The listing builds one solid part. Answer for the finished solid, in the listing's coordinates (mm). Face numbers are marked on the shaded views. A direction names the side the tool comes from. Coordinates: 2 decimals unless noted, no trailing zeros. Return JSON: item names as keys, results as strings. Group by question number.
1. Each of these flat-tipped pins is pushed along its axis until it touches: P1, Ø3, axis at x = -27.5, y = -23, coming from the +Z side; P2, Ø3, axis at x = -21, z = 20.5, coming from the +Y side; P3, Ø12, axis at x = 2.5, y = -15, coming from the -Z side; P4, Ø3, axis at x = 52, z = 13.5, coming from the +Y side. Where does it stop, or does it pass through?
2. The mould has two halves that part along X. Classify the marked faces 5, 6 and 7: pulls with the +X half, pulls with the -X half, needs draft (parallel to the pull), parting line crosses it, or undercut.
3. Which of the six approach directions +Z, -Z, +X, -X, +Y, -Y give full straight-line access (tool end or side, diameter ignored) to the marked faces 1, 2, 3 and 4?
4. Find the intervals of material crossed by line 1 along X through (y, z) = (-25, 13.25); line 2 along Y through (x, z) = (0, 20.65); line 3 along Z through (x, y) = (28, -15.75), in increasing order.
5. Section B-B (z = 21) is taken. State how many separate pieces and enclosed holes the cut face has, and give its area (3 significant figures).
```python
from build123d import *
from OCP.BRepFilletAPI import BRepFilletAPI_MakeChamfer

# Parameters (mm, degrees)
SKETCH1_R           = 2.675
SKETCH1_R_2         = 6.5
BOSS_EXTRUDE1_DEPTH = 26
CUT_EXTRUDE2_START  = 6
SKETCH1_4_R         = 11.05
SKETCH1_4_R_2       = 6.5
CUT_EXTRUDE2_DEPTH  = 8
SKETCH5_R           = 11.05
CUT_EXTRUDE6_DEPTH  = 6
CUT_EXTRUDE6_DRAFT  = 5
SKETCH4_R           = 5.25
CUT_EXTRUDE5_DEPTH  = 6.5
CUT_EXTRUDE10_START = -7
SKETCH9_R           = 11.05
CUT_EXTRUDE10_DEPTH = 7
CHAMFER5_SIZE       = 1.5
CHAMFER5_SIZE2      = 1.650094301
SKETCH6_R           = 2.75
CUT_EXTRUDE7_DEPTH  = 14
CUT_EXTRUDE8_START  = -7
SKETCH7_R           = 2.75
SKETCH7_W           = 8.1
SKETCH7_H           = 1.5
CUT_EXTRUDE8_DEPTH  = 4


with BuildPart() as part:
    # Sketch1 → Boss-Extrude1 (new body)
    with BuildSketch(Plane.XY):
        with BuildLine():
            Line((-37.5, -32.7), (60, -32.7))
            Line((60, -32.7), (60, -3))
            Line((60, -3), (45.025, -3))
            ThreePointArc((45.025, -3), (40, -8.025), (34.975, -3))
            Line((34.975, -3), (21.9089023, -3))
            ThreePointArc((21.9089023, -3), (18.537902988, -1.692744729), (16.929606323, 1.545454545))
            ThreePointArc((16.929606323, 1.545454545), (-0.242190945, 16.998274723), (-16.966764387, 1.0625))
            ThreePointArc((-16.966764387, 1.0625), (-21.667640892, -8.933034803), (-31.937438845, -13))
            Line((-31.937438845, -13), (-37.5, -13))
            Line((-37.5, -13), (-37.5, -32.7))
        make_face()
        with Locations(Location((-27.5, -23, 0), (0, 0, 180))):
            Circle(SKETCH1_R, mode=Mode.SUBTRACT)
        with Locations(Location((50, -23, 0), (0, 0, 180))):
            Circle(SKETCH1_R, mode=Mode.SUBTRACT)
        with Locations(Location((0, 0, 0), (0, 0, 180))):
            Circle(SKETCH1_R_2, mode=Mode.SUBTRACT)
        with Locations(Location((11.25, -23, 0), (0, 0, 180))):
            Circle(SKETCH1_R, mode=Mode.SUBTRACT)
    extrude(amount=BOSS_EXTRUDE1_DEPTH)

    # Sketch1<4> → Cut-Extrude2 (cut)
    with BuildSketch(Plane.XY.offset(CUT_EXTRUDE2_START)):
        Circle(SKETCH1_4_R)
        with Locations(Location((0, 0, 0), (0, 0, 180))):
            Circle(SKETCH1_4_R_2, mode=Mode.SUBTRACT)
    extrude(amount=CUT_EXTRUDE2_DEPTH, mode=Mode.SUBTRACT)


with BuildPart() as cut_extrude6_tool:
    # Sketch5 → Cut-Extrude6 (with draft: the straight prism first)
    with BuildSketch(Plane.XY.offset(6)):
        Circle(SKETCH5_R)
    extrude(amount=-CUT_EXTRUDE6_DEPTH)
    # Cut-Extrude6: the draft: its side faces are tilted about the plane it starts from
    cut_extrude6_sides = [cut_extrude6_tool.faces().sort_by_distance(p)[0] for p in [
        (-11.05, 0, 3),
    ]]
    draft(cut_extrude6_sides, Plane.XY.offset(6), CUT_EXTRUDE6_DRAFT)


with BuildPart() as part_1:
    add(part.part)

    # Cut-Extrude6: cut by cut_extrude6_tool
    add(cut_extrude6_tool.part, mode=Mode.SUBTRACT)

    # Sketch4 → Cut-Extrude5 (cut)
    with BuildSketch(Plane.XY.offset(26)):
        with Locations((-27.5, -23)):
            Circle(SKETCH4_R)
        with Locations((50, -23)):
            Circle(SKETCH4_R)
        with Locations((11.25, -23)):
            Circle(SKETCH4_R)
    extrude(amount=-CUT_EXTRUDE5_DEPTH, mode=Mode.SUBTRACT)

    # Sketch9 → Cut-Extrude10 (cut)
    with BuildSketch(Plane.XY.offset(26).offset(CUT_EXTRUDE10_START)):
        Circle(SKETCH9_R)
    extrude(amount=CUT_EXTRUDE10_DEPTH, mode=Mode.SUBTRACT)

    # Chamfer5: one chamfer whose edges measure the first distance from different faces: ONE call of the kernel's chamfer builder (chamfer() names one face for all edges)
    chamfer5_edges_1 = [part_1.edges().sort_by_distance(p)[0] for p in [
        (28.44195115, -3, 26),
        (18.537902988, -1.692744729, 26),
        (52.5125, -3, 0),
        (-34.718719423, -13, 0),
        (-21.667640892, -8.933034803, 0),
        (-0.242190945, 16.998274723, 0),
        (-0.242190945, 16.998274723, 26),
        (18.537902988, -1.692744729, 0),
        (28.44195115, -3, 0),
        (-21.667640892, -8.933034803, 26),
        (60, -3, 13),
        (60, -32.7, 13),
        (-37.5, -32.7, 13),
        (-37.5, -13, 13),
        (-34.718719423, -13, 26),
        (-37.5, -22.85, 26),
        (11.25, -32.7, 26),
        (60, -17.85, 26),
        (6.5, 0, 14),
        (52.5125, -3, 26),
        (-32.75, -23, 26),
        (44.75, -23, 26),
        (6, -23, 26),
        (6.5, 0, 19),
        (-11.05, 0, 26),
    ]]
    chamfer5_edges_2 = [part_1.edges().sort_by_distance(p)[0] for p in [
        (-11.574931981, 0, 0),
    ]]
    chamfer5_side_2 = [part_1.faces().sort_by_distance(p)[0] for p in [
        (12.610092139, -16.470965453, 0),
    ]]
    chamfer5 = BRepFilletAPI_MakeChamfer(part_1.part.solid().wrapped)
    for e in chamfer5_edges_1:
        chamfer5.Add(CHAMFER5_SIZE, e.wrapped)
    for e in chamfer5_edges_2:
        chamfer5.Add(CHAMFER5_SIZE, CHAMFER5_SIZE2, e.wrapped, chamfer5_side_2[0].wrapped)  # the first distance lies on this face
    add(Compound.cast(chamfer5.Shape()), mode=Mode.REPLACE)

    # Sketch6 → Cut-Extrude7 (cut)
    with BuildSketch(Plane(origin=(0, -3, 0), x_dir=(1, 0, 0), z_dir=(0, 1, 0))):
        with Locations(Location((52, -12.5, 0), (0, 0, 180))):
            Circle(SKETCH6_R)
        with Locations(Location((28, -12.5, 0), (0, 0, 180))):
            Circle(SKETCH6_R)
    extrude(amount=-CUT_EXTRUDE7_DEPTH, mode=Mode.SUBTRACT)

    # Sketch7 → Cut-Extrude8 (cut)
    # profile 1 of 5: a face of its own
    with BuildSketch(Plane(origin=(0, -3, 0), x_dir=(1, 0, 0), z_dir=(0, 1, 0)).offset(CUT_EXTRUDE8_START)):
        Polygon((23.95, -10.16173141), (23.95, -14.83826859), (28, -17.17653718), (32.05, -14.83826859), (32.05, -10.16173141), (28, -7.82346282), align=None)
        with Locations(Location((28, -12.5, 0), (0, 0, 180))):
            Circle(SKETCH7_R, mode=Mode.SUBTRACT)
    # profile 2 of 5: a face of its own
    with BuildSketch(Plane(origin=(0, -3, 0), x_dir=(1, 0, 0), z_dir=(0, 1, 0)).offset(CUT_EXTRUDE8_START)):
        Polygon((28, -17.17653718), (23.95, -14.83826859), (23.95, -24.5), (32.05, -24.5), (32.05, -14.83826859), align=None)
    # profile 3 of 5: a face of its own
    with BuildSketch(Plane(origin=(0, -3, 0), x_dir=(1, 0, 0), z_dir=(0, 1, 0)).offset(CUT_EXTRUDE8_START)):
        Polygon((47.95, -10.16173141), (47.95, -14.83826859), (52, -17.17653718), (56.05, -14.83826859), (56.05, -10.16173141), (52, -7.82346282), align=None)
    # profile 4 of 5: a face of its own
    with BuildSketch(Plane(origin=(0, -3, 0), x_dir=(1, 0, 0), z_dir=(0, 1, 0)).offset(CUT_EXTRUDE8_START)):
        Polygon((47.95, -26), (56.05, -26), (56.05, -14.83826859), (52, -17.17653718), (47.95, -14.83826859), align=None)
    # profile 5 of 5: a face of its own
    with BuildSketch(Plane(origin=(0, -3, 0), x_dir=(1, 0, 0), z_dir=(0, 1, 0)).offset(CUT_EXTRUDE8_START)):
        with Locations((28, -25.25)):
            Rectangle(SKETCH7_W, SKETCH7_H)
    extrude(amount=-CUT_EXTRUDE8_DEPTH, mode=Mode.SUBTRACT)


solid = part_1.part
```
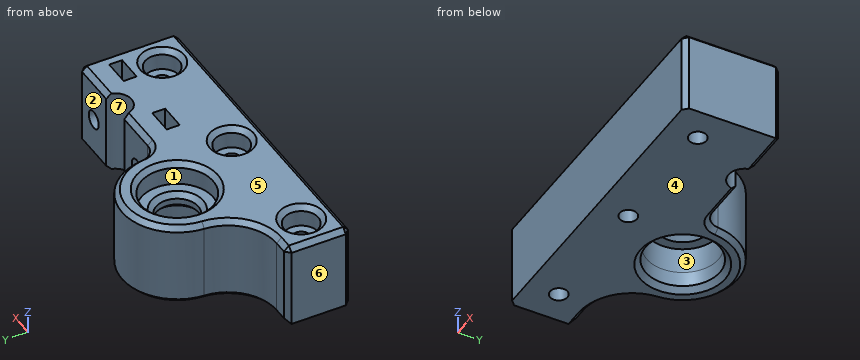
The answers:
{
 "1": {"P1": "passes through", "P2": "stops at y = -6.39", "P3": "stops at z = 0", "P4": "stops at y = -17"},
 "2": {"face 5": "needs draft", "face 6": "pulls with the -X half", "face 7": "undercut"},
 "3": {"face 1": "+Z", "face 2": "+Z, -Z, +X, +Y", "face 3": "-Z", "face 4": "-Z, +X, -X, +Y, -Y"},
 "4": {"line 1": "x = -37.5 to -29.28, -25.72 to 9.47, 13.03 to 48.22, 51.78 to 60", "line 2": "y = -32.7 to -11.05, 11.05 to 17", "line 3": "z = 0 to 9.75, 15.25 to 26"},
 "5": {"separate pieces": "1", "enclosed holes": "6", "area": "2,550 mm2"}
}
